Can you work these out from the model? Positions are in its coordinate system, mm. Face numbers are marked on the shaded views. A direction names the side the tool comes from. Give positions to 0.01 mm unless a question says otherwise; leave off trailing zeros. Loops run counter-clockwise (first coordinate to the right, second up) from the corner with the lowest first, then second, coordinate; pieces in that order, holes last. Notation, with made-up numbers: (2, -35.75) - (20, -35.75) arc R18 ccw to (20, -22.75) - close; hole circle Ø6 at (46, 33.5). An arc over 180 degrees is marked (long way). Answer in a Markdown table with one row per item.
from build123d import *

# Parameters (mm, degrees)
PAD_DEPTH       = 2
SKETCH001_R     = 3
POCKET_DEPTH    = 1
SKETCH002_R     = 1.75
POCKET001_DEPTH = 1
SKETCH003_W     = 2
SKETCH003_H     = 6
PAD001_DEPTH    = 4
SKETCH004_R     = 1.45
POCKET002_DEPTH = 3
SKETCH005_R     = 1.45
POCKET003_DEPTH = 3
FILLET_R        = 2.99
FILLET001_R     = 1
SKETCH006_W     = 12.25
SKETCH006_H     = 20
POCKET004_DEPTH = 2
SKETCH007_W     = 50.5
SKETCH007_H     = 12
PAD002_DEPTH    = 2
SKETCH008_W     = 50.5
SKETCH008_H     = 8
POCKET005_DEPTH = 2
FILLET002_R     = 1


with BuildPart() as part:
    # Sketch → Pad (new body)
    with BuildSketch(Plane.XY):
        Polygon((0, 0), (0, 29.5), (-1.25, 29.5), (-1.25, 89), (51.75, 89), (51.75, 29.5), (50.5, 29.5), (50.5, 0), align=None)
    extrude(amount=PAD_DEPTH)

    # Sketch001 (on Face10 of Pad) → Pocket (cut)
    with BuildSketch(Plane.XY.offset(2)):
        with Locations((2.75, 85)):
            Circle(SKETCH001_R)
        with Locations((47.75, 85)):
            Circle(SKETCH001_R)
    extrude(amount=-POCKET_DEPTH, mode=Mode.SUBTRACT)

    # Sketch002 (on Face13 of Pocket) → Pocket001 (cut)
    with BuildSketch(Plane.XY.offset(1)):
        with Locations((2.75, 85)):
            Circle(SKETCH002_R)
        with Locations((47.75, 85)):
            Circle(SKETCH002_R)
    extrude(amount=-POCKET001_DEPTH, mode=Mode.SUBTRACT)

    # Sketch003 (on Face5 of Pocket001) → Pad001 (join)
    with BuildSketch(Plane.XY.offset(2)):
        with Locations((1, 22)):
            Rectangle(SKETCH003_W, SKETCH003_H)
        with Locations((49.5, 22)):
            Rectangle(SKETCH003_W, SKETCH003_H)
    extrude(amount=PAD001_DEPTH)

    # Sketch004 (on Face6 of Pad001) → Pocket002 (cut)
    with BuildSketch(Plane(origin=(0, 0, 0), x_dir=(0, -1, 0), z_dir=(-1, 0, 0))):
        with Locations((-22, 3)):
            Circle(SKETCH004_R)
    extrude(amount=-POCKET002_DEPTH, mode=Mode.SUBTRACT)

    # Sketch005 (on Face25 of Pocket002) → Pocket003 (cut)
    with BuildSketch(Plane.YZ.offset(50.5)):
        with Locations((22, 3)):
            Circle(SKETCH005_R)
    extrude(amount=-POCKET003_DEPTH, mode=Mode.SUBTRACT)

    # Fillet
    fillet_edges = [part.edges().sort_by_distance(p)[0] for p in [
        (1, 25, 6),
        (1, 19, 6),
        (49.5, 19, 6),
        (49.5, 25, 6),
    ]]
    fillet(fillet_edges, radius=FILLET_R)

    # Fillet001
    fillet001_edges = [part.edges().sort_by_distance(p)[0] for p in [
        (2, 19.975, 2),
        (2, 24.025, 2),
        (48.5, 19.975, 2),
        (48.5, 24.025, 2),
    ]]
    fillet(fillet001_edges, radius=FILLET001_R)

    # Sketch006 (on Face5 of Fillet001) → Pocket004 (cut)
    with BuildSketch(Plane.XY.offset(2)):
        with Locations((9.875, 68)):
            Rectangle(SKETCH006_W, SKETCH006_H)
    extrude(amount=-POCKET004_DEPTH, mode=Mode.SUBTRACT)

    # Sketch007 (on Face32 of Pocket004) → Pad002 (join)
    with BuildSketch(Plane(origin=(0, 0, 0), x_dir=(1, 0, 0), z_dir=(0, 0, -1))):
        with Locations((25.25, -10)):
            Rectangle(SKETCH007_W, SKETCH007_H)
    extrude(amount=PAD002_DEPTH)

    # Sketch008 (on Face5 of Pad002) → Pocket005 (cut)
    with BuildSketch(Plane.XY.offset(2)):
        with Locations((25.25, 10)):
            Rectangle(SKETCH008_W, SKETCH008_H)
    extrude(amount=-POCKET005_DEPTH, mode=Mode.SUBTRACT)

    # Fillet002
    fillet002_edges = [part.edges().sort_by_distance(p)[0] for p in [
        (25.25, 14, 2),
        (25.25, 6, 2),
        (25.25, 16, -2),
        (25.25, 4, -2),
    ]]
    fillet(fillet002_edges, radius=FILLET002_R)


solid = part.part
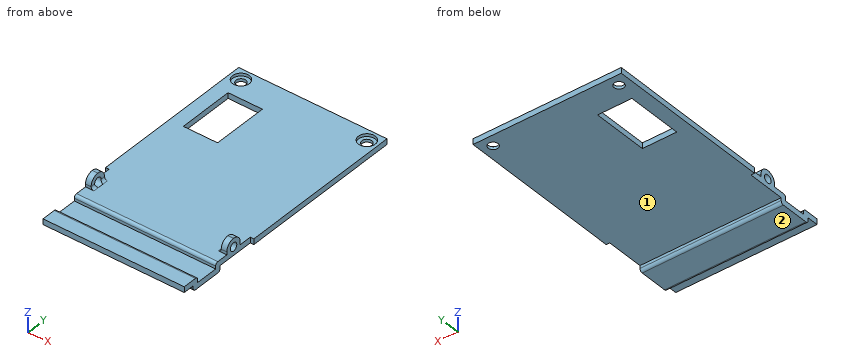
Q1. Imagine slicing it at C-C, the plane y = 52. Write out the boundary of the cut face in (x, z), and give its area (3 significant figures).
Checked values:
| item | result |
|---|---|
| outline | (-1.25, 0) - (51.75, 0) - (51.75, 2) - (-1.25, 2) - close |
| area | 106 mm² |
Q2. If I drill on line 1 (Y direction, x = 2.75, z = 0.55); line 2 (X direction, y = 85, z = 0.75); line 3 (Y direction, x = 0.65, z = 3), over which ranges is the centre line in solid material (lowest first)? Write a range as [from, to].
Checked values:
| item | result |
|---|---|
| line 1 | y = [0, 6], [14, 83.25], [86.75, 89] |
| line 2 | x = [-1.25, 1], [4.5, 46], [49.5, 51.75] |
| line 3 | y = [19, 20.55], [23.45, 25] |
Q3. Imagine slicing it at A-A, the plane y = 62.5. Write out the boundary of the cut face in (x, z).
Checked values:
| item | result |
|---|---|
| outline | (-1.25, 0) - (3.75, 0) - (3.75, 2) - (-1.25, 2) - close; (16, 0) - (51.75, 0) - (51.75, 2) - (16, 2) - close |
Q4. On a 3-axis mill with a long thin cutter (end or side, diameter ignored), from which of +Z, -Z, +X, -X, +Y, -Y can I reach the whole of each face in a straight line? I mean the marked faces 1 and 2. Say none if no direction works.
Checked values:
| item | result |
|---|---|
| face 1 | -Z, +X, -X, +Y |
| face 2 | -Z, +X, -X, +Y, -Y |
Q5. Imagine slicing it at B-B, the plane x = 11.5. Write out the boundary of the cut face in (y, z), and give its area (3 significant figures).
Checked values:
| item | result |
|---|---|
| outline | (0, 0) - (4, 0) - (4, -1) arc R1 ccw to (5, -2) - (15, -2) arc R1 ccw to (16, -1) - (16, 0) - (58, 0) - (58, 2) - (15, 2) arc R1 ccw to (14, 1) - (14, 0) - (6, 0) - (6, 1) arc R1 ccw to (5, 2) - (0, 2) - close; (78, 0) - (89, 0) - (89, 2) - (78, 2) - close |
| area | 145 mm² |
Q6. For pin 1 (2.5 mm diameter, centred on x = 13.5, y = 2, fed in from +Z); pin 2 (1.5 mm diameter, centred on x = 10.5, z = 2.5, fed in from -Y); pin 3 (5.5 mm diameter, centred on x = 2.75, y = 85, fed in from -Z); pin 4 (6.5 mm diameter, centred on x = 28.5, y = 11, fed in from +Z), each with a flat end and sliding along its axis, tell me the tip position at first contact or that it passes through.
Checked values:
| item | result |
|---|---|
| pin 1 | stops at z = 2 |
| pin 2 | stops at y = 0 |
| pin 3 | stops at z = 0 |
| pin 4 | stops at z = 1.66 |
